Autodesk Inventor part; units mm, degrees
ref_plane "YZ Plane" through (0, 0, 0) normal (1, 0, 0) x (0, 1, 0)
ref_plane "XZ Plane" through (0, 0, 0) normal (0, 1, 0) x (-1, 0, 0)
ref_plane "XY Plane" through (0, 0, 0) normal (0, 0, 1) x (1, 0, 0)
sketch "Sketch1" plane through (0, 0, 0) normal (0, 1, 0) x (-1, 0, 0)
  circle A0 centre (0, 0) radius 5
  dimension "d0" = 10
extrude "Extrusion1" add sketch "Sketch1" along normal blind 9
sketch "Sketch2" plane through (0, 9, 0) normal (0, 1, 0) x (1, 0, 0)
  circle A0 centre (0, 0) radius 3.5
  dimension "d3" = 7
extrude "Extrusion2" add sketch "Sketch2" along normal blind 5
sketch "Sketch3" plane through (0, 0, 0) normal (0, -1, 0) x (1, 0, 0)
  line L0 (8, 8) -> (-8, 8)
  line L1 (-8, 8) -> (-8, -8)
  line L2 (-8, -8) -> (8, -8)
  line L3 (8, -8) -> (8, 8)
  point P0 (0, 0)
  dimension "d6" = 16
  dimension "d7" = 16
  dimension "d8" = 8
  dimension "d9" = 8
extrude "Extrusion3" add sketch "Sketch3" along normal blind 2
chamfer "Chamfer1" distance 2 angle 45 4 edges at (-8, -2, 0) (0, -2, 8) (8, -2, 0) (0, -2, -8)
fillet "Fillet1" radius 2 4 edges at (7, -1.0001, 7.0001) (-7.0001, -1.0001, 7) (-7, -1.0001, -7.0001) (7.0001, -1.0001, -7)
sketch "Sketch4" plane through (0, -2, 0) normal (0, -1, 0) x (1, 0, 0)
  circle A0 centre (0, 0) radius 4.5
  dimension "d16" = 9
extrude "Extrusion4" add sketch "Sketch4" along normal blind 1.5
fillet "Fillet2" radius 0.2 1 edges at (-4.5, -3.5, 0)
sketch "Sketch5" plane through (0, 9, 0) normal (0, 1, 0) x (1, 0, 0)
  circle A0 centre (0, 0) radius 5
  line L0 (2.1794, -4.5) -> (-2.1794, -4.5)
  arc A1 (-2.1794, -4.5) -> (2.1794, -4.5) centre (0, 0) ccw
  dimension "d20" = 4.5
extrude "Extrusion5" cut sketch "Sketch5" against normal blind 9 contours L0 A0 picked at (-0.3727, -4.6245)
properties part number "StartBtn"
Could you check a few things on this model? Use its own coordinates, in mm. A direction names the side the tool comes from. Give positions to 0.01 mm unless a question says otherwise; leave off trailing zeros. Order: outer loops, then holes, each group sorted by start corner. A loop starts at its lowest first (then second) coordinate and runs counter-clockwise, first axis right, second up. Notation, with made-up numbers: M -4.5,80 L 38.5,80 A24 cw 38.5,95 Z; hole C 20,20.5 d11. An arc over 180 degrees is marked long. One line per question, with ' | ' between items.
1. I'm going to push flat-ended pins straight in: pin 1 (1.3 mm diameter, centred on x = -1, y = 3.5, fed in from +Z); pin 2 (1 mm diameter, centred on x = 5, z = -2.5, fed in from -Y); pin 3 (5 mm diameter, centred on y = 12, z = -3, fed in from +X). Where does each tip first touch, or does it pass through?
Results:
pin 1: z = 4.5 | pin 2: y = -2 | pin 3: x = 3.46
2. For faces 1 (the face through (0, -1, 7)), 2 (the face through (0, 5, 4.5)), 3 (the face through (3.233, 11.465, -1.341)), 4 (the face through (3, -2, 4)), 5 (the face through (0, 14, 0)), which set-ups out of +Z, -Z, +X, -X, +Y, -Y let a thin tool reach every point of the face, with its end or its side?
Results:
face 1: +Z, +X, -X, -Y | face 2: +Z, +X, -X, +Y | face 3: +Y | face 4: -Y | face 5: +Z, -Z, +X, -X, +Y
3. I want a section at C-C (y = 11). List the corners of the cut face in (x, z) for me.
Results:
outline: C 0,0 d7
4. If I drill on line 1 (Y direction, x = -5.5, z = -3); line 2 (Y direction, x = -1.25, z = -4); line 3 (X direction, y = 6.75, z = -1), over which ranges is the centre line in solid material (lowest first)?
Results:
line 1: -2 to 0 | line 2: -3.5 to 9 | line 3: -4.9 to 4.9
5. I want a section at D-D (y = 0.5). List the corners of the cut face in (x, z) for me.
Results:
outline: M -2.18,4.5 A5 ccw long 2.18,4.5 Z
